```python
from build123d import *

# Parameters (mm, degrees)
SKETCH2_W               = 90
SKETCH2_H               = 90
BOSS_EXTRUDE1_DEPTH     = 20
CUT_EXTRUDE1_DEPTH      = 67.708320321
CUT_EXTRUDE1_DEPTH_BACK = 67.708320321
CUT_EXTRUDE2_DEPTH      = 67.708320486
CUT_EXTRUDE2_DEPTH_BACK = 67.708320486
BOSS_EXTRUDE2_START     = 7.5
BOSS_EXTRUDE2_DEPTH     = 26
BOSS_EXTRUDE3_START     = 4
SKETCH6_W               = 3
SKETCH6_H               = 20
BOSS_EXTRUDE3_DEPTH     = 20
CUT_EXTRUDE3_START      = 30
CUT_EXTRUDE3_DEPTH      = 10


with BuildPart() as part:
    # Sketch2 → Boss-Extrude1 (new body)
    with BuildSketch(Plane.XY):
        Rectangle(SKETCH2_W, SKETCH2_H)
    extrude(amount=BOSS_EXTRUDE1_DEPTH)

    # Sketch3 → Cut-Extrude1 (cut, two sides)
    with BuildSketch(Plane(origin=(0, 0, 0), x_dir=(0, 0, -1), z_dir=(1, 0, 0))) as cut_extrude1_sk:
        with BuildLine():
            Line((0, -45), (0, 45))
            Line((0, 45), (-17.5, 45))
            add(Edge.make_bspline(
                [(-17.5, 45), (6.726056833, 3.093816892), (-17.5, -45)],
                knots=[0, 0, 0, 1, 1, 1], degree=2))
            Line((-17.5, -45), (0, -45))
        make_face()
        with BuildLine():
            add(Edge.make_bspline(
                [(-20, 45), (4.227639313, 5.03468062), (-20, -45)],
                knots=[0, 0, 0, 1, 1, 1], degree=2))
            Line((-20, -45), (-20, 45))
        make_face()
    extrude(amount=CUT_EXTRUDE1_DEPTH, mode=Mode.SUBTRACT)
    extrude(cut_extrude1_sk.sketch, amount=-CUT_EXTRUDE1_DEPTH_BACK, mode=Mode.SUBTRACT)

    # Sketch4 → Cut-Extrude2 (cut, two sides)
    with BuildSketch(Plane.XY) as cut_extrude2_sk:
        with BuildLine():
            Line((0, -41.973736842), (0, -45))
            Line((0, -45), (45, -45))
            Line((45, -45), (45, 45))
            Line((45, 45), (0, 45))
            add(Edge.make_bspline(
                [(17.375058461, -36.236668515), (37.115061452, -9.091765806), (61.513002786, 39.355563534), (0, 45)],
                knots=[0, 0, 0, 0, 1, 1, 1, 1], degree=3))
            ThreePointArc((17.375058461, -36.236668515), (12.021587761, -41.224158712), (7.425035075, -35.531495855))
            ThreePointArc((7.425035075, -35.531495855), (4.915119907, -40.138681352), (0, -41.973736842))
        make_face()
        with BuildLine():
            Line((-45, -45), (0, -45))
            Line((0, -45), (0, -41.973736842))
            ThreePointArc((0, -41.973736842), (-5.751088308, -39.287777066), (-7.382925452, -33.153732383))
            ThreePointArc((-7.382925452, -33.153732383), (-20.792123146, -43.404847745), (-32.187801105, -30.953724389))
            add(Edge.make_bspline(
                [(-32.187801105, -30.953724389), (-34.107884409, -0.978450852), (-64.097466043, 43.988968502), (-4.230485268, 45)],
                knots=[0, 0, 0, 0, 0.977737851, 0.977737851, 0.977737851, 0.977737851], degree=3))
            Line((-4.230485268, 45), (-45, 45))
            Line((-45, 45), (-45, -45))
        make_face()
        with BuildLine():
            ThreePointArc((-7.382925452, -33.153732383), (-5.751088308, -39.287777066), (0, -41.973736842))
            Line((0, -41.973736842), (0, -26.973736842))
            ThreePointArc((0, -26.973736842), (-4.814040224, -28.722648535), (-7.382925452, -33.153732383))
        make_face()
        with BuildLine():
            Line((0, -26.973736842), (0, -41.973736842))
            ThreePointArc((0, -41.973736842), (4.915119907, -40.138681352), (7.425035075, -35.531495855))
            ThreePointArc((7.425035075, -35.531495855), (7.481235295, -35.003942903), (7.5, -34.473736842))
            ThreePointArc((7.5, -34.473736842), (5.303300859, -29.170435983), (0, -26.973736842))
        make_face()
    extrude(amount=CUT_EXTRUDE2_DEPTH, mode=Mode.SUBTRACT)
    extrude(cut_extrude2_sk.sketch, amount=-CUT_EXTRUDE2_DEPTH_BACK, mode=Mode.SUBTRACT)

    # Sketch5 → Boss-Extrude2 (add)
    with BuildSketch(Plane.XY.offset(BOSS_EXTRUDE2_START)):
        Polygon((5.987927079, -17.143883964), (8.953511265, 2.40618792), (5.98744237, 2.856116036), (2.953607811, -17.143883964), align=None)
    extrude(amount=BOSS_EXTRUDE2_DEPTH)

    # Sketch6 → Boss-Extrude3 (add)
    with BuildSketch(Plane(origin=(0, 0, 0), x_dir=(0, 0, -1), z_dir=(1, 0, 0)).offset(BOSS_EXTRUDE3_START)):
        with Locations((-32, -7.143883964)):
            Rectangle(SKETCH6_W, SKETCH6_H)
    extrude(amount=BOSS_EXTRUDE3_DEPTH)

    # Sketch7 → Cut-Extrude3 (cut)
    with BuildSketch(Plane.XY.offset(CUT_EXTRUDE3_START)):
        Polygon((4, -10.245734651), (5.98744237, 2.856116036), (3.019616762, 2.856116036), (3.582073592, -13.000838136), align=None)
    extrude(amount=CUT_EXTRUDE3_DEPTH, mode=Mode.SUBTRACT)


solid = part.part
```
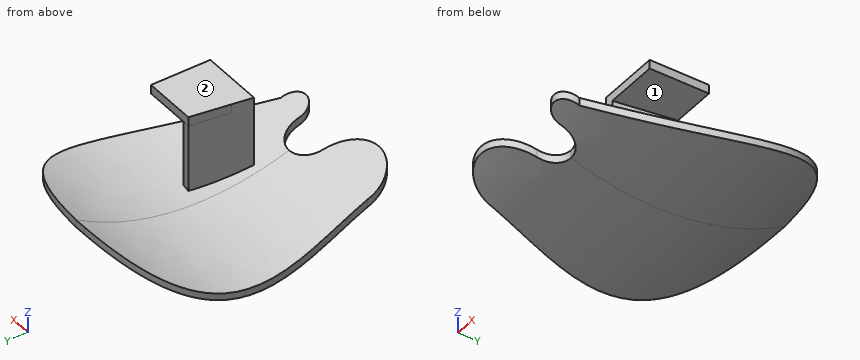
Model file for the job. Use its own axes, mm. Face numbers are marked on the shaded views. Coordinates: 2 decimals unless noted, no trailing zeros. Loops run counter-clockwise (first coordinate to the right, second up) from the corner with the lowest first, then second, coordinate; pieces in that order, holes last. Notation, with made-up numbers: (14, -14) - (38, -14) arc R23 cw to (38, 5) - close; hole circle Ø3 at (-11, -2.75). An arc over 180 degrees is marked (long way). Answer as a JSON object with one key per item and string values. Group by question number.
(1) Flat gauge pins, fed straight in: pin 1 (10 mm diameter, centred on y = 12, z = 9, fed in from -X); pin 2 (8 mm diameter, centred on y = -10.5, z = 25, fed in from -X); pin 3 (1.5 mm diameter, centred on y = -14.5, z = 26, fed in from +X). Where does each tip first touch, or does it go through?
(2) Probe line 1 along Y through (x, z) = (12, 32.25); line 2 along X through (y, z) = (-14, 18.5); line 3 along Z through (x, y) = (-36.5, 17). List the from-to ranges inside material, lowest first.
(3) Two-plate mould, pull along Z, no slides. Class the marked faces 1 and 2: released by +Z, released by -Z, zero draft, split by the parting line, or undercut.
(4) Cut at A-A (z = 22). Give the cut face in (x, y), then the cut area to 3 significant figures.
Geometry says:
{
 "1": {"pin 1": "stops at x = -41.36", "pin 2": "stops at x = 3.35", "pin 3": "stops at x = 6.5"},
 "2": {"line 1": "y = -17.14 to 2.86", "line 2": "x = 3.43 to 6.46", "line 3": "z = 6.85 to 9.19"},
 "3": {"face 1": "undercut", "face 2": "released by +Z"},
 "4": {"outline": "(2.95, -17.14) - (5.99, -17.14) - (8.95, 2.41) - (5.99, 2.86) - close", "area": "60.0 mm^2"}
}
